from build123d import *

# Parameters (mm, degrees)
F1_DEPTH = 38.1
F2_DEPTH = 12.7
F5_D     = 9.525
F6_D     = 9.525
F7_D     = 25.4


with BuildPart() as f1:
    # F0 (on Front) → F1 (new body)
    with BuildSketch(Plane.XZ):
        Polygon((0, 9.525), (0, 0), (127, 0), (127, 9.525), (101.6, 9.525), align=None)
    extrude(amount=F1_DEPTH)

    # F0 (on Front) → F2 (join)
    with BuildSketch(Plane.XZ):
        with BuildLine():
            Line((89.0406588905, 60.1776572782), (0, 9.525))
            Line((0, 9.525), (101.6, 9.525))
            Line((101.6, 9.525), (127, 9.525))
            Line((127, 9.525), (127, 38.1))
            ThreePointArc((127, 38.1), (114.3701357827, 60.0564029862), (89.0406588905, 60.1776572782))
        make_face()
    extrude(amount=F2_DEPTH)

    # F5 (through all)
    with Locations(Plane.XY.offset(9.525)):
        with Locations((25.3964494914, -25.3996793181)):
            Hole(F5_D / 2)

    # F6 (through all)
    with Locations(Plane.XY.offset(9.525)):
        with Locations((101.6, -25.4)):
            Hole(F6_D / 2)

    # F7 (through all)
    with Locations(Plane(origin=(0, 0, 0), x_dir=(1, 0, 0), z_dir=(0, 1, 0))):
        with Locations((101.6, -38.1)):
            Hole(F7_D / 2)


solid = f1.part
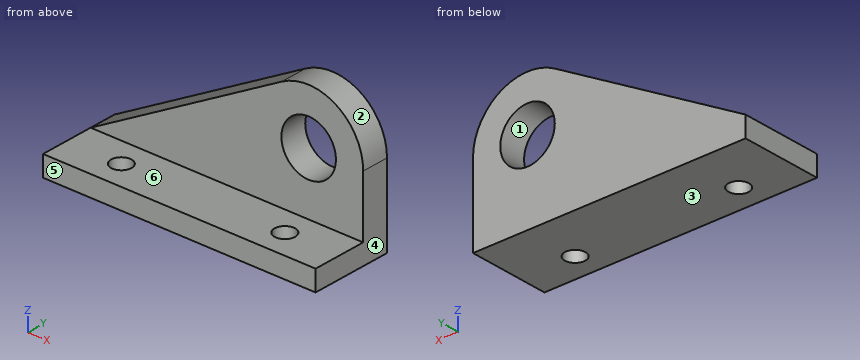
Could you check a few things on this model? Use its own coordinates, in mm. Face numbers are marked on the shaded views. A direction names the side the tool comes from. Coordinates: 2 decimals unless noted, no trailing zeros. Order: outer loops, then holes, each group sorted by start corner. A loop starts at its lowest first (then second) coordinate and runs counter-clockwise, first axis right, second up. Notation, with made-up numbers: (58.5, 57) -> (112.5, 57) arc R28 cw to (112.5, 96) -> close; hole circle Ø8 at (9, 87.5). An arc over 180 degrees is marked (long way). One line per question, with ' | ' between items.
Q1. Imagine slicing it at B-B on y = -9. Please give me the cut outline in (x, z) (3 decimals).
Return value:
outline: (0, 0) -> (127, 0) -> (127, 38.1) arc R25.4 ccw to (89.041, 60.178) -> (0, 9.525) -> close; hole circle Ø25.4 at (101.6, 38.1)
Q2. On a 3-axis mill with a long thin cutter (end or side, diameter ignored), from which of +Z, -Z, +X, -X, +Y, -Y can I reach the whole of each face in a straight line? I mean the marked faces 5 and 6. Say none if no direction works.
Return value:
face 5: +Z, -Z, +X, -X, -Y | face 6: +Z, +X, -X, -Y
Q3. If I drill on L1, parallel to X at y = -25, z = 5; L2, parallel to Y at x = 9, z = 14; L3, parallel to Z at x = 57, y = -29 (3 decimals), over which ranges is the centre line in solid material (lowest first)?
Return value:
L1: 0 to 20.65, 30.14 to 96.85, 106.35 to 127 | L2: -12.7 to 0 | L3: 0 to 9.525
Q4. Thinking about a two-plate mould opening in X: for the marked faces 1, 2, 3 and 4, which applies, pulls with the +X half, pulls with the -X half, needs draft (parallel to the pull), parting line crosses it, or undercut?
Return value:
face 1: undercut | face 2: parting line crosses it | face 3: needs draft | face 4: pulls with the +X half
Q5. Imagine slicing it at D-D on y = -22.5. Please give me the cut outline in (x, z) (3 decimals), and give its area (3 significant figures).
Return value:
outline: (0, 0) -> (21.618, 0) -> (21.618, 9.525) -> (0, 9.525) -> close; (29.174, 0) -> (97.822, 0) -> (97.822, 9.525) -> (29.174, 9.525) -> close; (105.378, 0) -> (127, 0) -> (127, 9.525) -> (105.378, 9.525) -> close | area: 1,070 mm²
Q6. Imagine slicing it at A-A on x = 101.6. Please give me the cut outline in (y, z) (1 decimal).
Return value:
outline: (-38.1, 0) -> (-30.2, 0) -> (-30.2, 9.5) -> (-38.1, 9.5) -> close; (-20.6, 0) -> (0, 0) -> (0, 25.4) -> (-12.7, 25.4) -> (-12.7, 9.5) -> (-20.6, 9.5) -> close; (-12.7, 50.8) -> (0, 50.8) -> (0, 63.5) -> (-12.7, 63.5) -> close
Q7. Imagine slicing it at C-C on z = 30.5. Please give me the cut outline in (x, y), and give its area (3 significant figures).
Return value:
outline: (36.87, -12.7) -> (91.43, -12.7) -> (91.43, 0) -> (36.87, 0) -> close; (111.77, -12.7) -> (127, -12.7) -> (127, 0) -> (111.77, 0) -> close | area: 886 mm²
Q8. I'm going to push flat-ended pins straight in: P1, Ø8, axis at x = 56.5, y = -33, coming from the +Z side (3 decimals); P2, Ø15, axis at x = 101.6, z = 38.1, coming from the -Y side; P3, Ø10, axis at x = 75, y = -12, coming from the +Z side; P4, Ø3, axis at x = 90, z = 26.5, coming from the -Y side. Where does each tip first touch, or does it pass through?
Return value:
P1: z = 9.525 | P2: through | P3: z = 55.03 | P4: y = -12.7
